Autodesk Inventor part; units mm, degrees
ref_plane "YZ Plane" through (0, 0, 0) normal (1, 0, 0) x (0, 1, 0)
ref_plane "XZ Plane" through (0, 0, 0) normal (0, 1, 0) x (-1, 0, 0)
ref_plane "XY Plane" through (0, 0, 0) normal (0, 0, 1) x (1, 0, 0)
sketch "Skizze1" plane through (0, 0, 0) normal (0, 0, 1) x (1, 0, 0)
  line L0 (0, 0) -> (45, 0)
  line L1 (45, 0) -> (45, 25)
  line L2 (45, 25) -> (0, 25)
  line L3 (0, 25) -> (0, 0)
  dimension "d5" = 45
  dimension "d6" = 25
extrude "Extrusion1" add sketch "Skizze1" along normal blind 2
sketch "Skizze3" plane through (0, 25, 0) normal (0, 1, 0) x (1, 0, 0)
  circle A0 centre (3.5, 8) radius 1.75
  circle A1 centre (41.5, 8) radius 1.75
  line L0 (3.5, 8) -> (41.5, 8) construction
  line L1 (0, 0) -> (45, 0) construction
  line L2 (22.5, 0) -> (22.5, 8) construction
  line L3 (0, 0) -> (7, 0)
  line L4 (45, 0) -> (38, 0)
  line L5 (0, 0) -> (0, 8)
  line L6 (7, 8) -> (7, 0)
  line L7 (38, 8) -> (38, 0)
  line L8 (45, 0) -> (45, 8)
  arc A2 (7, 8) -> (0, 8) centre (3.5, 8) ccw
  arc A3 (45, 8) -> (38, 8) centre (41.5, 8) ccw
  dimension "d2" = 38
  dimension "d3" = 3.5
  dimension "d4" = 8
extrude "Extrusion2" add sketch "Skizze3" against normal up to surface (25 mm away)
sketch "Skizze4" plane through (0, 0, 2) normal (0, 0, 1) x (1, 0, 0)
  line L0 (3.45, 5.261) -> (41.55, 5.261) construction
  line L1 (41.55, 5.261) -> (41.55, 19.739) construction
  line L2 (41.55, 19.739) -> (3.45, 19.739) construction
  line L3 (3.45, 19.739) -> (3.45, 5.261) construction
  line L4 (45, 25) -> (0, 25) construction
  line L5 (22.5, 25) -> (22.5, 0) construction
  line L6 (0, 0) -> (45, 0) construction
  line L7 (0, 25) -> (0, 0) construction
  line L8 (0, 12.5) -> (45, 12.5) construction
  line L9 (45, 0) -> (45, 25) construction
  circle A0 centre (41.55, 19.739) radius 1.5
  circle A1 centre (3.45, 5.261) radius 1.5
  point P0 (22.5, 19.739)
  point P1 (41.55, 12.5)
  dimension "d12" = 38.1
  dimension "d13" = 14.478
  dimension "d14" = 3
extrude "Extrusion3" cut sketch "Skizze4" against normal blind 8
sketch "Skizze5" plane through (0, 0, 2) normal (0, 0, 1) x (1, 0, 0)
  line L0 (44.09, 22.4949) -> (0.91, 22.4949) construction
  line L1 (0.91, 22.4949) -> (0.91, 2.5051) construction
  line L2 (0.91, 2.5051) -> (44.09, 2.5051) construction
  line L3 (44.09, 2.5051) -> (44.09, 22.4949) construction
  line L4 (45, 25) -> (0, 25) construction
  line L5 (22.5, 25) -> (22.5, 0) construction
  line L6 (0, 0) -> (45, 0) construction
  line L7 (45, 0) -> (45, 25) construction
  line L8 (45, 12.5) -> (0, 12.5) construction
  line L9 (0, 25) -> (0, 0) construction
  line L10 (15, 6.0051) -> (30, 6.0051)
  line L11 (30, 6.0051) -> (30, 2.0051)
  line L12 (30, 2.0051) -> (15, 2.0051)
  line L13 (15, 2.0051) -> (15, 6.0051)
  point P0 (0.91, 12.5)
  point P1 (22.5, 6.0051)
  dimension "d17" = 43.18
  dimension "d18" = 19.9898
  dimension "d19" = 15
  dimension "d20" = 4
  dimension "d27" = 0.5
extrude "Extrusion4" cut sketch "Skizze5" against normal up to next
fillet "Rundung1" radius 1 4 edges at (15, 6.0051, 1) (30, 6.0051, 1) (30, 2.0051, 1) (15, 2.0051, 1)
fillet "Rundung2" radius 4 2 edges at (7, 12.5, 0) (38, 12.5, 0)
fillet "Rundung3" radius 1 2 edges at (0, 12.5, 2) (45, 12.5, 2)
properties part number "US Halterung hinten" material "ABS-Kunststoff"
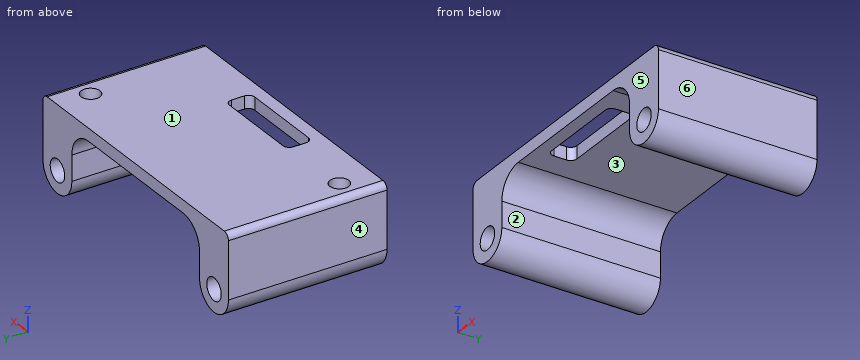
Here's how the part is built. I have some questions about the finished solid (model axes, mm). Face numbers are marked on the shaded views. A direction names the side the tool comes from. Coordinates: 2 decimals unless noted, no trailing zeros. Write each loop counter-clockwise with the first axis right and the second up, starting at its lowest first coordinate (ties: lowest second). Pieces come first, ordered by that corner, then holes.
Item 1: I want a section at B-B on y = 9.5. Write out the boundary of the cut face in (x, z).
Item 2: I want a section at D-D on z = -7. Write out the boundary of the cut face in (x, y), and give its area (3 significant figures).
Item 3: If we mould it in two halves opening along X, with no side actions, what happens to the marked faces 3, 4, 5 and 6? For each: +X half, -X half, draft (parallel to the pull), parting line (faces both ways), or undercut.
Item 4: I want a section at A-A on z = -4.75. Write out the boundary of the cut face in (x, y).
Item 5: If I drill on line 1 (X direction, y = 11.5, z = -8); line 2 (Y direction, x = 3.45, z = -3.75); line 3 (Y direction, x = 22, z = 0.5), over which ranges is the centre line in solid material (lowest first)?
Item 6: On a 3-axis mill with a long thin cutter (end or side, diameter ignored), from which of +Z, -Z, +X, -X, +Y, -Y can I reach the whole of each face in a straight line? I mean the marked faces 1 and 2. Say none if no direction works.
Item 7: Will these pins go through, and if not, where does the flat tip stop? pin 1 (2.5 mm diameter, centred on x = 3.45, y = 5.261, fed in from +Z); pin 2 (1 mm diameter, centred on x = 9, y = 10, fed in from -Z); pin 3 (12 mm diameter, centred on x = 17, y = 22, fed in from -Z).
Item 8: I want a section at C-C on x = 3.45. Write out the boundary of the cut face in (y, z), and give its area (3 significant figures).
Findings below:
1. outline: (0, -8) arc R3.5 ccw to (7, -8) - (7, -4) arc R4 cw to (11, 0) - (34, 0) arc R4 cw to (38, -4) - (38, -8) arc R3.5 ccw to (45, -8) - (45, 1) arc R1 ccw to (44, 2) - (1, 2) arc R1 ccw to (0, 1) - close; hole circle Ø3.5 at (3.5, -8); hole circle Ø3.5 at (41.5, -8)
2. outline: (0, 0) - (2.06, 0) - (2.06, 25) - (0, 25) - close; (4.94, 0) - (7, 0) - (7, 25) - (4.94, 25) - close; (38, 0) - (40.06, 0) - (40.06, 25) - (38, 25) - close; (42.94, 0) - (45, 0) - (45, 25) - (42.94, 25) - close
2. area: 206 mm2
3. face 3: undercut
3. face 4: -X half
3. face 5: draft
3. face 6: +X half
4. outline: (0, 0) - (7, 0) - (7, 25) - (0, 25) - close; (38, 0) - (45, 0) - (45, 25) - (38, 25) - close; hole circle Ø3 at (3.45, 5.26); hole circle Ø3 at (41.55, 19.74)
5. line 1: x = 0 to 1.75, 5.25 to 7, 38 to 39.75, 43.25 to 45
5. line 2: y = 0 to 3.76, 6.76 to 25
5. line 3: y = 0 to 2.01, 6.01 to 25
6. face 1: +Z, +X, -X, +Y, -Y
6. face 2: -Z, +Y, -Y
7. pin 1: stops at z = -6
7. pin 2: stops at z = -0.88
7. pin 3: stops at z = 0
8. outline: (0, -11.5) - (25, -11.5) - (25, -9.75) - (0, -9.75) - close; (0, -6.25) - (25, -6.25) - (25, 2) - (6.76, 2) - (6.76, -6) - (3.76, -6) - (3.76, 2) - (0, 2) - close
8. area: 226 mm2
